Could you check a few things on this model? Use its own coordinates, in mm. A direction names the side the tool comes from. Coordinates: 2 decimals unless noted, no trailing zeros. Order: outer loops, then holes, each group sorted by start corner. A loop starts at its lowest first (then second) coordinate and runs counter-clockwise, first axis right, second up. Notation, with made-up numbers: (60.25, 69.25) -> (80.25, 69.25) arc R25 cw to (80.25, 81.25) -> close; hole circle Ø9 at (-9.5, 44.5). An arc over 180 degrees is marked (long way). Put each result on its own line as item: value. Start each with the question number.
Q1. If we section it at A-A (x = 12.5): Please give me the cut outline in (y, z) (1 decimal), and give its area (3 significant figures).
Q2. If we section it at B-B (z = -7.5): Please give me the cut outline in (x, y) (1 decimal).
Q3. For faces 4 (the face through (1, 9.525, -13)), 5 (the face through (0, 3, -6)), 6 (the face through (12, 5.08, -4)), which set-ups out of +Z, -Z, +X, -X, +Y, -Y let a thin tool reach every point of the face, with its end or its side?
Q4. If we section it at D-D (x = 41): Please give me the cut outline in (y, z) (1 decimal).
Q5. If we section it at C-C (y = 27): Please give me the cut outline in (x, z) (1 decimal).
Q6. Please list where these lines run through material, in increasing order: line 1 along Y through (x, z) = (45, -4.25); line 2 along X through (y, z) = (48, -7.75); line 3 along Y through (x, z) = (9, -6.25).
Q7. Will these pins go through, and if not, where does the flat tip stop? pin 1 (24 mm diameter, centred on x = 37, y = 35.5, fed in from -Z); pin 2 (0.5 mm diameter, centred on y = 48.5, z = -13.5, fed in from -X); pin 3 (1 mm diameter, centred on x = 1, z = -13.5, fed in from -Y).
Q8. We'd pull the mould along X, two halves only. Please class faces 1 (the face through (0, 8, -13)), 2 (the face through (1, 22.86, -13)), 3 (the face through (37, 2.54, -7)): +X half, -X half, draft (parallel to the pull), parting line (faces both ways), or undercut.
from build123d import *

# Parameters (mm, degrees)
SKETCH1_W                                         = 52.3875
SKETCH1_H                                         = 50.8
BOSS_EXTRUDE1_DEPTH                               = 1.905
SKETCH2_W                                         = 14.605
SKETCH2_H                                         = 50.8
BOSS_EXTRUDE2_DEPTH                               = 1.5875
BOSS_EXTRUDE3_DEPTH                               = 12.7
CUT_EXTRUDE1_REACH                                = 76.07
SKETCH4_W                                         = 10.16
SKETCH4_H                                         = 3.8608
CUT_EXTRUDE2_REACH                                = 76.07
SKETCH5_W                                         = 6.985
SKETCH5_H                                         = 12.7
SKETCH5_W_2                                       = 7.112
SKETCH6_W                                         = 10.16
SKETCH6_H                                         = 2.54
BOSS_EXTRUDE4_DEPTH                               = 8.8392
SKETCH8_W                                         = 1.27
SKETCH8_H                                         = 41.402
BOSS_EXTRUDE5_DEPTH                               = 14.2875
BOSS_EXTRUDE6_DEPTH                               = 1.5875
CUT_EXTRUDE3_REACH                                = 75.47
SKETCH11_W                                        = 1.5875
SKETCH11_H                                        = 5.08
CSK_FOR_4_FLAT_HEAD_MACHINE_SCREW_100_D           = 3.2639
CSK_FOR_4_FLAT_HEAD_MACHINE_SCREW_100_DEPTH       = 7.493
CSK_FOR_4_FLAT_HEAD_MACHINE_SCREW_100_CSINK_D     = 5.715
CSK_FOR_4_FLAT_HEAD_MACHINE_SCREW_100_CSINK_ANGLE = 100
CSK_FOR_4_FLAT_HEAD_MACHINE_SCREW_100_TIP         = 0.980574487


with BuildPart() as part:
    # Sketch1 → Boss-Extrude1 (new body)
    with BuildSketch(Plane.XY):
        with Locations((26.19375, 25.4)):
            Rectangle(SKETCH1_W, SKETCH1_H)
    extrude(amount=BOSS_EXTRUDE1_DEPTH)

    # Sketch2 → Boss-Extrude2 (add)
    with BuildSketch(Plane.ZY):
        with Locations((-5.3975, 25.4)):
            Rectangle(SKETCH2_W, SKETCH2_H)
    extrude(amount=BOSS_EXTRUDE2_DEPTH)

    # Sketch3 → Boss-Extrude3 (add)
    with BuildSketch(Plane(origin=(0, 0, 0), x_dir=(-1, 0, 0), z_dir=(0, 0, -1))):
        Polygon((0, 50.8), (-52.3875, 50.8), (-52.3875, 0), (0, 0), (0, 2.54), (-49.8475, 2.54), (-49.8475, 48.26), (0, 48.26), align=None)
    extrude(amount=BOSS_EXTRUDE3_DEPTH)

    # Sketch4 → Cut-Extrude1 (cut, up to next)
    with BuildSketch(Plane.XZ, mode=Mode.PRIVATE) as cut_extrude1_sk1:
        with Locations((12.065, -10.7696)):
            Rectangle(SKETCH4_W, SKETCH4_H)
    cut_extrude1_tool1 = extrude(cut_extrude1_sk1.sketch, amount=-CUT_EXTRUDE1_REACH, mode=Mode.PRIVATE) & part.part
    add(cut_extrude1_tool1.solids().sort_by_distance((12.065, 0, -10.7696))[0], mode=Mode.SUBTRACT)

    # Sketch5 → Cut-Extrude2 (cut, up to next)
    with BuildSketch(Plane.XZ, mode=Mode.PRIVATE) as cut_extrude2_sk1:
        with Locations((3.4925, -6.35)):
            Rectangle(SKETCH5_W, SKETCH5_H)
    cut_extrude2_tool1 = extrude(cut_extrude2_sk1.sketch, amount=-CUT_EXTRUDE2_REACH, mode=Mode.PRIVATE) & part.part
    # Sketch5 → Cut-Extrude2 (cut, up to next)
    with BuildSketch(Plane.XZ, mode=Mode.PRIVATE) as cut_extrude2_sk2:
        with Locations((20.701, -6.35)):
            Rectangle(SKETCH5_W_2, SKETCH5_H)
    cut_extrude2_tool2 = extrude(cut_extrude2_sk2.sketch, amount=-CUT_EXTRUDE2_REACH, mode=Mode.PRIVATE) & part.part
    add(cut_extrude2_tool1.solids().sort_by_distance((3.4925, 0, -6.35))[0], mode=Mode.SUBTRACT)
    add(cut_extrude2_tool2.solids().sort_by_distance((20.701, 0, -6.35))[0], mode=Mode.SUBTRACT)

    # Sketch6 → Boss-Extrude4 (add)
    with BuildSketch(Plane(origin=(0, 0, 0), x_dir=(-1, 0, 0), z_dir=(0, 0, -1))):
        with Locations((-12.065, 3.81)):
            Rectangle(SKETCH6_W, SKETCH6_H)
    extrude(amount=BOSS_EXTRUDE4_DEPTH)

    # Sketch8 → Boss-Extrude5 (add)
    with BuildSketch(Plane(origin=(0, 0, 0), x_dir=(-1, 0, 0), z_dir=(0, 0, -1))):
        with Locations((-0.635, 27.559)):
            Rectangle(SKETCH8_W, SKETCH8_H)
    extrude(amount=BOSS_EXTRUDE5_DEPTH)

    # Sketch9 → Boss-Extrude6 (add)
    with BuildSketch(Plane(origin=(0, 0, -12.7), x_dir=(-1, 0, 0), z_dir=(0, 0, -1))):
        Polygon((0, 48.26), (0, 48.895), (-50.4825, 48.895), (-50.4825, 1.905), (-24.257, 1.905), (-24.257, 2.54), (-49.8475, 2.54), (-49.8475, 48.26), align=None)
    extrude(amount=BOSS_EXTRUDE6_DEPTH)

    # Sketch11 → Cut-Extrude3 (cut, up to next)
    with BuildSketch(Plane(origin=(1.27, 0, 0), x_dir=(0, 0, -1), z_dir=(1, 0, 0)), mode=Mode.PRIVATE) as cut_extrude3_sk1:
        with Locations((13.49375, 25.4)):
            Rectangle(SKETCH11_W, SKETCH11_H)
    cut_extrude3_tool1 = extrude(cut_extrude3_sk1.sketch, amount=-CUT_EXTRUDE3_REACH, mode=Mode.PRIVATE) & part.part
    # Sketch11 → Cut-Extrude3 (cut, up to next)
    with BuildSketch(Plane(origin=(1.27, 0, 0), x_dir=(0, 0, -1), z_dir=(1, 0, 0)), mode=Mode.PRIVATE) as cut_extrude3_sk2:
        with Locations((13.49375, 12.065)):
            Rectangle(SKETCH11_W, SKETCH11_H)
    cut_extrude3_tool2 = extrude(cut_extrude3_sk2.sketch, amount=-CUT_EXTRUDE3_REACH, mode=Mode.PRIVATE) & part.part
    # Sketch11 → Cut-Extrude3 (cut, up to next)
    with BuildSketch(Plane(origin=(1.27, 0, 0), x_dir=(0, 0, -1), z_dir=(1, 0, 0)), mode=Mode.PRIVATE) as cut_extrude3_sk3:
        with Locations((13.49375, 46.355)):
            Rectangle(SKETCH11_W, SKETCH11_H)
    cut_extrude3_tool3 = extrude(cut_extrude3_sk3.sketch, amount=-CUT_EXTRUDE3_REACH, mode=Mode.PRIVATE) & part.part
    add(cut_extrude3_tool1.solids().sort_by_distance((1.27, 25.4, -13.49375))[0], mode=Mode.SUBTRACT)
    add(cut_extrude3_tool2.solids().sort_by_distance((1.27, 12.065, -13.49375))[0], mode=Mode.SUBTRACT)
    add(cut_extrude3_tool3.solids().sort_by_distance((1.27, 46.355, -13.49375))[0], mode=Mode.SUBTRACT)

    # CSK for #4 Flat Head Machine Screw (100)1
    with Locations(Plane.XY.offset(1.905)):
        with Locations((23.4188, 38.4175), (23.4188, 17.4625)):
            CounterSinkHole(CSK_FOR_4_FLAT_HEAD_MACHINE_SCREW_100_D / 2, CSK_FOR_4_FLAT_HEAD_MACHINE_SCREW_100_CSINK_D / 2, depth=CSK_FOR_4_FLAT_HEAD_MACHINE_SCREW_100_DEPTH, counter_sink_angle=CSK_FOR_4_FLAT_HEAD_MACHINE_SCREW_100_CSINK_ANGLE)
            with Locations((0, 0, -(CSK_FOR_4_FLAT_HEAD_MACHINE_SCREW_100_DEPTH + CSK_FOR_4_FLAT_HEAD_MACHINE_SCREW_100_TIP / 2))):  # 118° drill point
                Cone(0, CSK_FOR_4_FLAT_HEAD_MACHINE_SCREW_100_D / 2, CSK_FOR_4_FLAT_HEAD_MACHINE_SCREW_100_TIP, mode=Mode.SUBTRACT)


solid = part.part
The answers:
1. outline: (0, -8.8) -> (5.1, -8.8) -> (5.1, 0) -> (48.3, 0) -> (48.3, -14.3) -> (48.9, -14.3) -> (48.9, -12.7) -> (50.8, -12.7) -> (50.8, 1.9) -> (0, 1.9) -> close
1. area: 175 mm^2
2. outline: (-1.6, 0) -> (0, 0) -> (0, 6.9) -> (1.3, 6.9) -> (1.3, 48.3) -> (49.8, 48.3) -> (49.8, 2.5) -> (24.3, 2.5) -> (24.3, 0) -> (52.4, 0) -> (52.4, 50.8) -> (-1.6, 50.8) -> close; (7, 0) -> (17.1, 0) -> (17.1, 5.1) -> (7, 5.1) -> close
3. face 4: -Z, -X
3. face 5: -Z, -Y
3. face 6: -Z
4. outline: (0, -12.7) -> (1.9, -12.7) -> (1.9, -14.3) -> (2.5, -14.3) -> (2.5, 0) -> (48.3, 0) -> (48.3, -14.3) -> (48.9, -14.3) -> (48.9, -12.7) -> (50.8, -12.7) -> (50.8, 1.9) -> (0, 1.9) -> close
5. outline: (-1.6, -12.7) -> (1.3, -12.7) -> (1.3, 0) -> (49.8, 0) -> (49.8, -14.3) -> (50.5, -14.3) -> (50.5, -12.7) -> (52.4, -12.7) -> (52.4, 1.9) -> (-1.6, 1.9) -> close
6. line 1: 0 to 2.54, 48.26 to 50.8
6. line 2: -1.59 to 1.27, 49.85 to 52.39
6. line 3: 0 to 5.08, 48.26 to 50.8
7. pin 1: z = 0
7. pin 2: x = 1.27
7. pin 3: y = 6.86
8. face 1: -X half
8. face 2: draft
8. face 3: undercut
